Read the model definition and answer for the solid it produces. Units are mm, in the model's axes. Coordinates: 2 decimals unless noted, no trailing zeros. Order: outer loops, then holes, each group sorted by start corner. A loop starts at its lowest first (then second) coordinate and runs counter-clockwise, first axis right, second up.
```python
from build123d import *

# Parameters (mm, degrees)
ESQUISSE1_W             = 5.5
ESQUISSE1_H             = 7.5
BOSS_EXTRU_1_DEPTH      = 80
CONG_1_R                = 3.5
CONG_2_R                = 2
ESQUISSE2_R             = 0.7
ENL_V_MAT_EXTRU_1_DEPTH = 81.276475384


with BuildPart() as part:
    # Esquisse1 → Boss.-Extru.1 (new body)
    with BuildSketch(Plane.XY):
        Rectangle(ESQUISSE1_W, ESQUISSE1_H)
    extrude(amount=BOSS_EXTRU_1_DEPTH)

    # Congé1
    # the kernel refuses this fillet: 3.5 mm, written as the material it takes off along each edge
    with BuildSketch(Plane(origin=(-2.75, 3.75, -8.75), x_dir=(1, 0, 0), z_dir=(0, 0, 1))) as cong_1_piece_1:
        with BuildLine():
            CenterArc((CONG_1_R, -CONG_1_R), CONG_1_R, 90, 90)
            Line((0, -CONG_1_R), (0, 0))
            Line((0, 0), (CONG_1_R, 0))
        make_face()
    extrude(amount=97.5, mode=Mode.SUBTRACT)
    with BuildSketch(Plane(origin=(2.75, 3.75, -8.75), x_dir=(-1, 0, 0), z_dir=(0, 0, 1))) as cong_1_piece_2:
        with BuildLine():
            CenterArc((CONG_1_R, CONG_1_R), CONG_1_R, 180, 90)
            Line((0, CONG_1_R), (0, 0))
            Line((0, 0), (CONG_1_R, 0))
        make_face()
    extrude(amount=97.5, mode=Mode.SUBTRACT)

    # Congé2
    cong_2_edges = [part.edges().sort_by_distance(p)[0] for p in [
        (2.75, -3.75, 40),
        (-2.75, -3.75, 40),
    ]]
    fillet(cong_2_edges, radius=CONG_2_R)

    # Esquisse2 → Enlèv. mat.-Extru.1 (cut, through all)
    with BuildSketch(Plane.ZY.offset(2.75)):
        with Locations(Location((46, 0, 0), (0, 0, 159.075167572))):
            Circle(ESQUISSE2_R)
        with Locations(Location((51, 0, 0), (0, 0, 159.075167572))):
            Circle(ESQUISSE2_R)
        with Locations(Location((56, 0, 0), (0, 0, 159.075167572))):
            Circle(ESQUISSE2_R)
        with Locations(Location((61, 0, 0), (0, 0, 159.075167572))):
            Circle(ESQUISSE2_R)
        with Locations(Location((66, 0, 0), (0, 0, 159.075167572))):
            Circle(ESQUISSE2_R)
        with Locations(Location((71, 0, 0), (0, 0, 159.075167572))):
            Circle(ESQUISSE2_R)
        with Locations(Location((76, 0, 0), (0, 0, 159.075167572))):
            Circle(ESQUISSE2_R)
    extrude(amount=-ENL_V_MAT_EXTRU_1_DEPTH, mode=Mode.SUBTRACT)


solid = part.part
```
1) A flat-ended cylindrical pin translates along its axis: pin 1 Ø1.5 at (y, z) = (1.5, 21.5) entering from -X. Find the tip coordinate at first contact, or state that the pin passes through.
A:
pin 1: stops at x = -2.71
2) A cutting plane is placed at A-A, the plane z = 13.5. Determine the outline of the cut face in (x, y).
A:
outline: (-2.75, -1.75) arc R2 ccw to (-0.75, -3.75) - (0.75, -3.75) arc R2 ccw to (2.75, -1.75) - (2.75, 0.25) arc R3.5 ccw to (0, 3.67) arc R3.5 ccw to (-2.75, 0.25) - close
3) A cutting plane is placed at C-C, the plane x = 1.4. Determine the outline of the cut face in (y, z).
A:
outline: (-3.64, 0) - (3.01, 0) - (3.01, 80) - (-3.64, 80) - close; hole circle Ø1.4 at (0, 46); hole circle Ø1.4 at (0, 51); hole circle Ø1.4 at (0, 56); hole circle Ø1.4 at (0, 61); hole circle Ø1.4 at (0, 66); hole circle Ø1.4 at (0, 71); hole circle Ø1.4 at (0, 76)
4) Determine the mould class of faces 1 (the flat face through (0, 0, 80)), 2 (the flat face through (-2.75, -1, 39)), 3 (the cylindrical face through (-0.04, -0.28, 76.64)), 4 (the cylindrical face through (-0.04, -0.28, 71.64)) for opening direction Z: pulls with the +Z half, pulls with the -Z half, needs draft (parallel to the pull), parting line crosses it, or undercut.
A:
face 1: pulls with the +Z half
face 2: needs draft
face 3: undercut
face 4: undercut
5) A cutting plane is placed at B-B, the plane z = 71. Determine the outline of the cut face in (x, y).
A:
outline: (-2.75, -1.75) arc R2 ccw to (-0.75, -3.75) - (0.75, -3.75) arc R2 ccw to (2.75, -1.75) - (2.75, -0.7) - (-2.75, -0.7) - close; (-2.72, 0.7) - (2.72, 0.7) arc R3.5 ccw to (0, 3.67) arc R3.5 ccw to start
6) Straight lines are drawn through the part: line 1 (Y direction, x = -1, z = 56); line 2 (Y direction, x = -0.1, z = 60.5); line 3 (X direction, y = 0.5, z = 74.5). For each, find the intervals that lie inside material, in ascending order.
A:
line 1: y = -3.73 to -0.7, 0.7 to 3.28
line 2: y = -3.75 to -0.49, 0.49 to 3.65
line 3: x = -2.74 to 2.74
7) A cutting plane is placed at D-D, the plane x = -1.95. Determine the outline of the cut face in (y, z).
A:
outline: (-3.35, 0) - (2.48, 0) - (2.48, 80) - (-3.35, 80) - close; hole circle Ø1.4 at (0, 46); hole circle Ø1.4 at (0, 51); hole circle Ø1.4 at (0, 56); hole circle Ø1.4 at (0, 61); hole circle Ø1.4 at (0, 66); hole circle Ø1.4 at (0, 71); hole circle Ø1.4 at (0, 76)
